Geometry: final body of the model. Coordinates: model frame, mm. Face numbers are marked on the shaded views. Give positions to 0.01 mm unless a question says otherwise; leave off trailing zeros. Order: outer loops, then holes, each group sorted by start corner. A loop starts at its lowest first (then second) coordinate and runs counter-clockwise, first axis right, second up. Notation, with made-up numbers: (-22, 61) -> (28, 61) arc R10 cw to (28, 75) -> close; hole circle Ø8 at (60.25, 1). An arc over 180 degrees is marked (long way). One line per question, with ' | ' between items.
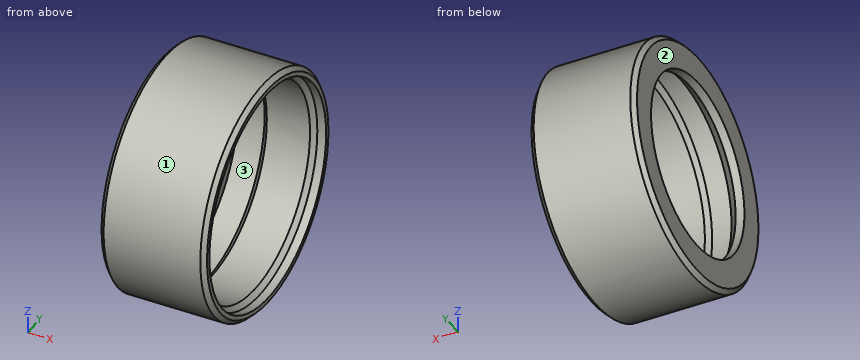
Autodesk Inventor part; units mm, degrees
ref_plane "YZ Plane" through (0, 0, 0) normal (1, 0, 0) x (0, 1, 0)
ref_plane "XZ Plane" through (0, 0, 0) normal (0, 1, 0) x (-1, 0, 0)
ref_plane "XY Plane" through (0, 0, 0) normal (0, 0, 1) x (1, 0, 0)
sketch "Skizze1" plane through (0, 0, 0) normal (0, 0, 1) x (1, 0, 0)
  line L0 (-14.4, 0) -> (2.4, 0)
  line L1 (0, -2.7) -> (0, 16.2)
  line L2 (0, 12.5) -> (-1, 12.5)
  line L3 (-1, 12.5) -> (-2, 11.5)
  line L4 (-2, 11.5) -> (-6, 11.5)
  line L5 (-6, 11.5) -> (-7, 12.5)
  line L6 (-7, 12.5) -> (-10, 12.5)
  line L7 (-10, 12.5) -> (-10, 11)
  line L8 (-0.5, 13.5) -> (-11.5, 13.5)
  line L9 (-12, 13) -> (-12, 10)
  line L10 (-12, 10) -> (-11, 10)
  line L11 (-11, 10) -> (-10, 11)
  line L12 (-11.5, 13.5) -> (-12, 13)
  line L13 (0, 13) -> (0, 12.5)
  line L14 (0, 13) -> (-0.5, 13.5)
  point P0 (0, 0)
  point P1 (0, 13.5)
  point P2 (-12, 13.5)
  dimension "d0" = 23
  dimension "d1" = 25
  dimension "d2" = 45
  dimension "d3" = 45
  dimension "d4" = 1
  dimension "d5" = 10
  dimension "d6" = 3
  dimension "d7" = 12
  dimension "d9" = 20
  dimension "d10" = 1
  dimension "d11" = 0.5
  dimension "d12" = 0.5
  dimension "d13" = 0.5
  dimension "d14" = 0.5
  dimension "d25" = 22
  dimension "d26" = 1
revolve "Umdrehung1" add sketch "Skizze1" angle 360 about axis through (-10, 0, 0) along (1, 0, 0)
hole "Bohrung1" at (0, 0, 0) direction (-1, 0, 0) diameter 23.917 depth 8
properties part number "13_0204_034"
1) Material intervals for probe 1 along Z at (x, y) = (-2.9, 0); probe 2 along Z at (x, y) = (-0.75, 0); probe 3 along Y at (x, z) = (-0.75, 11), sorted ascending. Write a range as from..to.
Check result:
probe 1: z = -13.5..-11.96, 11.96..13.5 | probe 2: z = -13.5..-12.5, 12.5..13.5 | probe 3: y = -7.83..-5.94, 5.94..7.83
2) Section C-C on x = -4. Return loops of the section in (y, z).
Check result:
outline: circle Ø27 at (0, 0); hole circle Ø23.92 at (0, 0)
3) Contact query for flat-ended pins moving along their axis: pin 1 Ø2 at (x, z) = (-8, -4) entering from -Y; pin 2 Ø16 at (y, z) = (0, 0) entering from -X; pin 3 Ø6 at (x, z) = (-3, 6.5) entering from +Y; pin 4 Ø6 at (x, y) = (-6, 5) entering from +Z. Output: stop coordinate, or through.
Check result:
pin 1: stops at y = -13.16 | pin 2: passes through | pin 3: stops at y = 13.04 | pin 4: stops at z = 13.35
4) Section A-A on z = 0. Return loops of the section in (x, y), plus the area to 3 significant figures.
Check result:
outline: (-12, -13) -> (-11.5, -13.5) -> (-0.5, -13.5) -> (0, -13) -> (0, -12.5) -> (-1, -12.5) -> (-1.54, -11.96) -> (-6.46, -11.96) -> (-7, -12.5) -> (-10, -12.5) -> (-10, -11) -> (-11, -10) -> (-12, -10) -> close; (-12, 10) -> (-11, 10) -> (-10, 11) -> (-10, 12.5) -> (-7, 12.5) -> (-6.46, 11.96) -> (-1.54, 11.96) -> (-1, 12.5) -> (0, 12.5) -> (0, 13) -> (-0.5, 13.5) -> (-11.5, 13.5) -> (-12, 13) -> close | area: 38.4 mm^2
5) Pull-direction query (Z, two-part tool) for the marked faces 1, 2 and 3; classes: +Z half, -Z half, draft (parallel to the pull), parting line (faces both ways), or undercut.
Check result:
face 1: parting line | face 2: draft | face 3: undercut
